Geometry check sheet. Reference: the model listing, model coordinates, mm. A direction names the side the tool comes from. Give positions to 0.01 mm unless a question says otherwise; leave off trailing zeros. Write each loop counter-clockwise with the first axis right and the second up, starting at its lowest first coordinate (ties: lowest second). Pieces come first, ordered by that corner, then holes. Notation, with made-up numbers: M 89.5,-14 L 144.5,-14 A18 cw 144.5,9 Z; hole C -9,6.25 d8. An arc over 180 degrees is marked long. One line per item, written item: value. Start each with the question number.
1. Cross-section at A-A on z = 0. Record the cut outline in (x, y).
2. Cross-section at D-D on y = -5.5. Record the cut outline in (x, z).
3. Release check for a two-part mould opening along Z. For faces 1 (the face through (-10, 4, -4)), 2 (the face through (-4.945, 6.783, -1.898)), 3 (the face through (3.94, 3.88, 9.35)), 4 (the face through (3.94, 5.65, -10.46)) record: pulls with the +Z half, pulls with the -Z half, needs draft (parallel to the pull), parting line crosses it, or undercut.
4. Cross-section at C-C on x = -1. Record the cut outline in (y, z).
5. Scan lines: line 1 (X direction, y = 7.85, z = 0); line 2 (Y direction, x = -2.5, z = -3.5); line 3 (Y direction, x = 2.25, z = 12). Record each from-to range of solid material in increasing order.
6. Cross-section at B-B on y = 0. Record the cut outline in (x, z).
7. Gauge pin test, flat ends, axial feed: pin 1 (2 mm diameter, centred on x = -5, y = 7, fed in from +Z); pin 2 (6 mm diameter, centred on x = 6, y = -7.5, fed in from -Z); pin 3 (3 mm diameter, centred on x = -2, z = -6, fed in from -Y); pin 4 (3.5 mm diameter, centred on x = -5.03, z = 0, fed in from -Y). Record the tip position at first contact, or that the pin passes through.
8. Tool access check on faces 5 (the face through (3.9, 11.4, 3.4)), 6 (the face through (3.94, -1.24, -11.87)), 7 (the face through (3.944, -10.124, 0.011)), 8 (the face through (3.94, 1.24, 11.87)), 9 (the face through (3.944, 10.49, -5.684)). Record the directions out of +Z, -Z, +X, -X, +Y, -Y that give a thin tool (end or side, any length) a straight path to the whole face; none if there is none.
from build123d import *

# Parameters (mm, degrees)
BASPROSKE_W              = 8
BASPROSKE_H              = 13.5
TOOTHCUT_DEPTH           = 21.700241544
TEETHCUTS_COUNT          = 16
TEETHCUTS_ANGLE          = 337.5
HUBNEAONESKE_R           = 9
HUBNEARONE_DEPTH         = 10.0000508
BORSKE_R                 = 5
BORE_DEPTH               = 18.0000508
CUT_EXTRUDE_1_DEPTH      = 22.308194049
CUT_EXTRUDE_1_DEPTH_BACK = 22.308194049
SKETCH_1_R               = 1.9


with BuildPart() as part:
    # BasProSke → Base-Revolve (revolve)
    with BuildSketch(Plane(origin=(0, 0, 0), x_dir=(1, 0, 0), z_dir=(0, 1, 0)), mode=Mode.PRIVATE) as base_revolve_sk:
        with Locations((4, 6.75)):
            Rectangle(BASPROSKE_W, BASPROSKE_H)
    revolve(base_revolve_sk.sketch.rotate(Axis((-10, 0, 0), (1, 0, 0)), 180), axis=Axis((-10, 0, 0), (1, 0, 0)))

    # TooCutSke → ToothCut (cut, through all)
    with BuildSketch(Plane(origin=(0, 0, 0), x_dir=(0, 0, -1), z_dir=(1, 0, 0))):
        with BuildLine():
            ThreePointArc((0.779807897, 10.093922708), (0, 10.124), (-0.779807897, 10.093922708))
            ThreePointArc((-0.779807897, 10.093922708), (-1.232785697, 11.858156262), (-2.310463203, 13.326597651))
            ThreePointArc((-2.310463203, 13.326597651), (0, 13.5254), (2.310463203, 13.326597651))
            ThreePointArc((2.310463203, 13.326597651), (1.232785697, 11.858156262), (0.779807897, 10.093922708))
        make_face()
    toothcut = extrude(amount=TOOTHCUT_DEPTH, mode=Mode.SUBTRACT)

    # TeethCuts: ToothCut ×16 about axis
    teethcuts_axis = Axis((-10, 0, 0), (1, 0, 0))
    for i in range(1, TEETHCUTS_COUNT):
        add(toothcut.rotate(teethcuts_axis, i * TEETHCUTS_ANGLE / (TEETHCUTS_COUNT - 1)), mode=Mode.SUBTRACT)

    # HubNeaOneSke → HubNearOne (add)
    with BuildSketch(Plane.ZY):
        with Locations(Location((0, 0, 0), (0, 0, 180))):
            Circle(HUBNEAONESKE_R)
    extrude(amount=HUBNEARONE_DEPTH)

    # BorSke → Bore (cut, symmetric)
    with BuildSketch(Plane(origin=(0, 0, 0), x_dir=(0, 0, -1), z_dir=(1, 0, 0))):
        with Locations(Location((0, 0, 0), (0, 0, 180))):
            Circle(BORSKE_R)
    extrude(amount=BORE_DEPTH, both=True, mode=Mode.SUBTRACT)

    # 草图1 → 切除-拉伸1 (cut, two sides: drawn at the far end of the back side and taken through both)
    with BuildSketch(Plane(origin=(0, 0, 0), x_dir=(1, 0, 0), z_dir=(0, 1, 0)).offset(-CUT_EXTRUDE_1_DEPTH_BACK)):
        with Locations(Location((-5.028528168, 0, 0), (0, 0, 270))):
            Circle(SKETCH_1_R)
    extrude(amount=CUT_EXTRUDE_1_DEPTH + CUT_EXTRUDE_1_DEPTH_BACK, mode=Mode.SUBTRACT)


solid = part.part
Report:
1. outline: M -10,-9 L -6.93,-9 L -6.93,-5 L -10,-5 Z; M -10,5 L -6.93,5 L -6.93,9 L -10,9 Z; M -3.13,-9 L 0,-9 L 0,-10.12 L 8,-10.12 L 8,-5 L -3.13,-5 Z; M -3.13,5 L 8,5 L 8,10.12 L 0,10.12 L 0,9 L -3.13,9 Z
2. outline: M -10,-7.12 L 0,-7.12 L 0,-10.32 L 8,-10.32 L 8,10.32 L 0,10.32 L 0,7.12 L -10,7.12 Z; hole C -5.03,0 d3.8
3. face 1: needs draft
3. face 2: undercut
3. face 3: undercut
3. face 4: pulls with the -Z half
4. outline: C 0,0 d18; hole C 0,0 d10
5. line 1: x = -10 to -6.93, -3.13 to 8
5. line 2: y = -8.29 to -3.57, 3.57 to 8.29
5. line 3: y = -3.34 to -1.3, 1.3 to 3.34
6. outline: M -10,-9 L 0,-9 L 0,-10.12 L 8,-10.12 L 8,-5 L -10,-5 Z; M -10,5 L 8,5 L 8,10.12 L 0,10.12 L 0,9 L -10,9 Z
7. pin 1: stops at z = 6.71
7. pin 2: stops at z = -11.42
7. pin 3: stops at y = -7.79
7. pin 4: passes through
8. face 5: +X, -X
8. face 6: -Z, +X, -X
8. face 7: +X, -X, -Y
8. face 8: +Z, +X, -X
8. face 9: +X, -X, +Y
